Autodesk Inventor part; units mm, degrees
ref_plane "YZ Plane" through (0, 0, 0) normal (1, 0, 0) x (0, 1, 0)
ref_plane "XZ Plane" through (0, 0, 0) normal (0, 1, 0) x (-1, 0, 0)
ref_plane "XY Plane" through (0, 0, 0) normal (0, 0, 1) x (1, 0, 0)
sketch "Sketch1" plane through (0, 0, 0) normal (0, 1, 0) x (-1, 0, 0)
  line L0 (200, 750) -> (-200, 750)
  line L1 (-200, 750) -> (-200, -750)
  line L2 (-200, -750) -> (200, -750)
  line L3 (200, -750) -> (200, 750)
  line L4 (200, 0) -> (-200, 0) construction
  line L5 (0, -750) -> (0, 750) construction
  point P0 (0, 0)
  point P1 (0, 0)
  dimension "d0" = 1500
  dimension "d1" = 400
extrude "Extrusion1" add sketch "Sketch1" along normal blind 350
sketch "Sketch2" plane through (200, 0, -750) normal (0, 0, -1) x (-1, 0, 0)
  line L0 (200, 0) -> (200, 350) construction
  line L1 (400, 350) -> (0, 350) construction
  line L2 (400, 0) -> (400, 350) construction
  line L3 (400, 175) -> (0, 175) construction
  line L4 (0, 0) -> (0, 350) construction
  circle A0 centre (200, 175) radius 100
  dimension "d4" = 200
extrude "Extrusion2" add sketch "Sketch2" along normal blind 350
sketch "Sketch3" plane through (0, 175, -1100) normal (0, 0, -1) x (-1, 0, 0)
  line L0 (-200, 175) -> (200, 175) construction
  line L1 (0, 175) -> (0, -175) construction
  circle A0 centre (0, 0) radius 100 construction
  circle A1 centre (0, 0) radius 250
  dimension "d7" = 500
extrude "Extrusion3" add sketch "Sketch3" along normal blind 200
fillet "Fillet1" radius 100 4 edges at (200, 350, 0) (-200, 350, 0) (200, 0, 0) (-200, 0, 0)
properties part number "car suspension wheel joint"
Here's how the part is built. I have some questions about the finished solid (model axes, mm). A direction names the side the tool comes from. Give positions to 0.01 mm unless a question says otherwise; leave off trailing zeros. Write each loop counter-clockwise with the first axis right and the second up, starting at its lowest first coordinate (ties: lowest second). Pieces come first, ordered by that corner, then holes. Notation, with made-up numbers: (12.25, -22) -> (58.25, -22) arc R22 cw to (58.25, 8) -> close; hole circle Ø6 at (20.5, 80). An arc over 180 degrees is marked (long way). Use one line per item in the form item = value. Start each with the question number.
1. On a 3-axis mill with a long thin cutter (end or side, diameter ignored), from which of +Z, -Z, +X, -X, +Y, -Y can I reach the whole of each face in a straight line? I mean faces 1 (the face through (200, 174, 10)), 2 (the face through (-200, 174, -10)), 3 (the face through (1, 0, 10)), 4 (the face through (1, 350, 10)), 5 (the face through (169.929, 321.484, -10.5)). Say none if no direction works.
2. Thinking about a two-plate mould opening in Z: for faces 6 (the face through (-3, 173, 750)), 7 (the face through (-169.929, 321.484, 10.5)), 8 (the face through (92, 134, -750)), 9 (the face through (21.68, 272.62, -922.55)), which applies, +Z half, -Z half, draft (parallel to the pull), parting line (faces both ways), or undercut?
3. Will these pins go through, and if not, where does the flat tip stop? pin 1 Ø2 at (x, z) = (-99, -607) entering from +Y; pin 2 Ø3 at (x, z) = (-17.5, -278) entering from -Y; pin 3 Ø1 at (y, z) = (124, -182.5) entering from +X.
4. If I drill on L1, parallel to Z at x = -109, y = 275.5; L2, parallel to Z at x = 171, y = 351.5; L3, parallel to X at y = 171, z = -18, over which ranges is the centre line in solid material (lowest first)?
5. Imagine slicing it at A-A on y = 175. List the corners of the cut face in (x, z) for me.
6. Imagine slicing it at C-C on x = -173.5. List the corners of the cut face in (y, z) for me, plus the area to 3 significant figures.
7. Imagine slicing it at B-B on x = 0. List the corners of the cut face in (y, z) for me.
8. Imagine slicing it at D-D on y = 52. List the corners of the cut face in (x, z) for me.
Entries:
q1.face_1 = +Z, +X, +Y, -Y
q1.face_2 = +Z, -X, +Y, -Y
q1.face_3 = +Z, +X, -X, -Y
q1.face_4 = +Z, +X, -X, +Y
q1.face_5 = +Z, +X, +Y
q2.face_6 = +Z half
q2.face_7 = draft
q2.face_8 = undercut
q2.face_9 = undercut
q3.pin_1 = 350
q3.pin_2 = 0
q3.pin_3 = 200
q4.L1 = -1300 to -1100, -750 to 750
q4.L2 = -1300 to -1100
q4.L3 = -200 to 200
q5.outline = (-250, -1300) -> (250, -1300) -> (250, -1100) -> (100, -1100) -> (100, -750) -> (200, -750) -> (200, 750) -> (-200, 750) -> (-200, -750) -> (-100, -750) -> (-100, -1100) -> (-250, -1100) -> close
q6.outline = (-4.99, -1300) -> (354.99, -1300) -> (354.99, -1100) -> (-4.99, -1100) -> close; (32.19, -750) -> (317.81, -750) -> (317.81, 750) -> (32.19, 750) -> close
q6.area = 500,000 mm²
q7.outline = (-75, -1300) -> (425, -1300) -> (425, -1100) -> (275, -1100) -> (275, -750) -> (350, -750) -> (350, 750) -> (0, 750) -> (0, -750) -> (75, -750) -> (75, -1100) -> (-75, -1100) -> close
q8.outline = (-217.65, -1300) -> (217.65, -1300) -> (217.65, -1100) -> (-217.65, -1100) -> close; (-187.73, -750) -> (187.73, -750) -> (187.73, 750) -> (-187.73, 750) -> close
